Work out the finished part from the listing and answer in its coordinate system (mm). Face numbers are marked on the shaded views. A direction names the side the tool comes from. Give positions to 0.01 mm unless a question says otherwise; leave off trailing zeros. Loops run counter-clockwise (first coordinate to the right, second up) from the corner with the lowest first, then second, coordinate; pieces in that order, holes last. Notation, with made-up numbers: (14.25, 59.25) - (41.25, 59.25) arc R23 ccw to (41.25, 70.25) - close; hole circle Ø10 at (59.25, -8.5). An arc over 180 degrees is marked (long way). One line per question, with ' | ' between items. Start each with the question number.
1. For a pull along Z with two mould halves and no side action, classify the marked faces 6, 7 and 8 as released by +Z, released by -Z, zero draft, split by the parting line, or undercut.
2. Which of the six approach directions +Z, -Z, +X, -X, +Y, -Y give full straight-line access (tool end or side, diameter ignored) to the marked faces 1, 2, 3, 4 and 5?
3. Find the intervals of material crossed by line 1 (Z direction, x = 2, y = 0.5); line 2 (X direction, y = 0.6, z = 2); line 3 (Z direction, x = 37.5, y = -0.25), in increasing order.
4. Section B-B (y = 3.25) is taken. Determine the outline of the cut face in (x, z).
5. Section A-A (z = 10) is taken. Determine the outline of the cut face in (x, y).
6. Each of these flat-tipped pins is pushed along its axis until it touches: pin 1 (12 mm diameter, centred on x = 41.5, z = 11.5, fed in from -Y); pin 2 (1.5 mm diameter, centred on y = 1.5, z = 7.5, fed in from +X); pin 3 (0.7 mm diameter, centred on x = 16.5, y = -6, fed in from +Z); pin 4 (2 mm diameter, centred on x = 25.5, z = 1, fed in from -Y). Where does it stop, or does it pass through?
7. Section C-C (y = -4.25) is taken. Give the number of separate pieces and of enclosed holes in the cut face, plus the area to 3 significant figures.
from build123d import *

# Parameters (mm, degrees)
SKETCH1_W           = 48.3
SKETCH1_H           = 25.5
SKETCH1_R           = 1.5
BOSS_EXTRUDE1_DEPTH = 4.4
FILLET1_R           = 2
SKETCH2_W           = 2.54
SKETCH2_H           = 2.54
BOSS_EXTRUDE2_DEPTH = 2.35
SKETCH3_W           = 0.66
SKETCH3_H           = 0.66
BOSS_EXTRUDE3_DEPTH = 5.33
SKETCH4_W           = 3.4
SKETCH4_H           = 7.5
CUT_EXTRUDE1_DEPTH  = 0.7
SKETCH5_W           = 7.5
SKETCH5_H           = 3.7
BOSS_EXTRUDE4_DEPTH = 0.3
SKETCH6_W           = 7.4
SKETCH6_H           = 16.14
CUT_EXTRUDE2_DEPTH  = 2.4
SKETCH7_W           = 4
SKETCH7_H           = 4
CUT_EXTRUDE3_DEPTH  = 3.3


with BuildPart() as part:
    # Sketch1 → Boss-Extrude1 (new body)
    with BuildSketch(Plane(origin=(0, 0, 0), x_dir=(1, 0, 0), z_dir=(0, 1, 0))):
        with Locations((24.15, -12.75)):
            Rectangle(SKETCH1_W, SKETCH1_H)
        with Locations((46.3, -2)):
            Circle(SKETCH1_R, mode=Mode.SUBTRACT)
        with Locations((2, -2)):
            Circle(SKETCH1_R, mode=Mode.SUBTRACT)
        with Locations((46.3, -23.5)):
            Circle(SKETCH1_R, mode=Mode.SUBTRACT)
        with Locations((2, -23.5)):
            Circle(SKETCH1_R, mode=Mode.SUBTRACT)
    extrude(amount=BOSS_EXTRUDE1_DEPTH)

    # Fillet1
    fillet1_edges = [part.edges().sort_by_distance(p)[0] for p in [
        (48.3, 2.2, 25.5),
        (0, 2.2, 25.5),
        (0, 2.2, 0),
        (48.3, 2.2, 0),
    ]]
    fillet(fillet1_edges, radius=FILLET1_R)

    # Sketch2 → Boss-Extrude2 (add)
    with BuildSketch(Plane.XZ):
        with Locations((6.37, 24.23)):
            Rectangle(SKETCH2_W, SKETCH2_H)
        with Locations((8.91, 24.23)):
            Rectangle(SKETCH2_W, SKETCH2_H)
        with Locations((11.45, 24.23)):
            Rectangle(SKETCH2_W, SKETCH2_H)
        with Locations((13.99, 24.23)):
            Rectangle(SKETCH2_W, SKETCH2_H)
        with Locations((16.53, 24.23)):
            Rectangle(SKETCH2_W, SKETCH2_H)
        with Locations((19.07, 24.23)):
            Rectangle(SKETCH2_W, SKETCH2_H)
        with Locations((21.61, 24.23)):
            Rectangle(SKETCH2_W, SKETCH2_H)
        with Locations((24.15, 24.23)):
            Rectangle(SKETCH2_W, SKETCH2_H)
        with Locations((26.69, 24.23)):
            Rectangle(SKETCH2_W, SKETCH2_H)
        with Locations((29.23, 24.23)):
            Rectangle(SKETCH2_W, SKETCH2_H)
        with Locations((31.77, 24.23)):
            Rectangle(SKETCH2_W, SKETCH2_H)
        with Locations((34.31, 24.23)):
            Rectangle(SKETCH2_W, SKETCH2_H)
        with Locations((36.85, 24.23)):
            Rectangle(SKETCH2_W, SKETCH2_H)
        with Locations((39.39, 24.23)):
            Rectangle(SKETCH2_W, SKETCH2_H)
        with Locations((41.93, 24.23)):
            Rectangle(SKETCH2_W, SKETCH2_H)
        with Locations((41.93, 1.27)):
            Rectangle(SKETCH2_W, SKETCH2_H)
        with Locations((39.39, 1.27)):
            Rectangle(SKETCH2_W, SKETCH2_H)
        with Locations((36.85, 1.27)):
            Rectangle(SKETCH2_W, SKETCH2_H)
        with Locations((34.31, 1.27)):
            Rectangle(SKETCH2_W, SKETCH2_H)
        with Locations((31.77, 1.27)):
            Rectangle(SKETCH2_W, SKETCH2_H)
        with Locations((29.23, 1.27)):
            Rectangle(SKETCH2_W, SKETCH2_H)
        with Locations((26.69, 1.27)):
            Rectangle(SKETCH2_W, SKETCH2_H)
        with Locations((24.15, 1.27)):
            Rectangle(SKETCH2_W, SKETCH2_H)
        with Locations((21.61, 1.27)):
            Rectangle(SKETCH2_W, SKETCH2_H)
        with Locations((19.07, 1.27)):
            Rectangle(SKETCH2_W, SKETCH2_H)
        with Locations((16.53, 1.27)):
            Rectangle(SKETCH2_W, SKETCH2_H)
        with Locations((13.99, 1.27)):
            Rectangle(SKETCH2_W, SKETCH2_H)
        with Locations((11.45, 1.27)):
            Rectangle(SKETCH2_W, SKETCH2_H)
        with Locations((8.91, 1.27)):
            Rectangle(SKETCH2_W, SKETCH2_H)
        with Locations((6.37, 1.27)):
            Rectangle(SKETCH2_W, SKETCH2_H)
    extrude(amount=BOSS_EXTRUDE2_DEPTH)

    # Sketch3 → Boss-Extrude3 (add)
    with BuildSketch(Plane.XZ.offset(2.35)):
        with Locations((6.37, 24.23)):
            Rectangle(SKETCH3_W, SKETCH3_H)
        with Locations((8.91, 24.23)):
            Rectangle(SKETCH3_W, SKETCH3_H)
        with Locations((11.45, 24.23)):
            Rectangle(SKETCH3_W, SKETCH3_H)
        with Locations((13.99, 24.23)):
            Rectangle(SKETCH3_W, SKETCH3_H)
        with Locations((16.53, 24.23)):
            Rectangle(SKETCH3_W, SKETCH3_H)
        with Locations((19.07, 24.23)):
            Rectangle(SKETCH3_W, SKETCH3_H)
        with Locations((21.61, 24.23)):
            Rectangle(SKETCH3_W, SKETCH3_H)
        with Locations((24.15, 24.23)):
            Rectangle(SKETCH3_W, SKETCH3_H)
        with Locations((26.69, 24.23)):
            Rectangle(SKETCH3_W, SKETCH3_H)
        with Locations((29.23, 24.23)):
            Rectangle(SKETCH3_W, SKETCH3_H)
        with Locations((31.77, 24.23)):
            Rectangle(SKETCH3_W, SKETCH3_H)
        with Locations((34.31, 24.23)):
            Rectangle(SKETCH3_W, SKETCH3_H)
        with Locations((36.85, 24.23)):
            Rectangle(SKETCH3_W, SKETCH3_H)
        with Locations((39.39, 24.23)):
            Rectangle(SKETCH3_W, SKETCH3_H)
        with Locations((41.93, 24.23)):
            Rectangle(SKETCH3_W, SKETCH3_H)
        with Locations((41.93, 1.27)):
            Rectangle(SKETCH3_W, SKETCH3_H)
        with Locations((39.39, 1.27)):
            Rectangle(SKETCH3_W, SKETCH3_H)
        with Locations((36.85, 1.27)):
            Rectangle(SKETCH3_W, SKETCH3_H)
        with Locations((34.31, 1.27)):
            Rectangle(SKETCH3_W, SKETCH3_H)
        with Locations((31.77, 1.27)):
            Rectangle(SKETCH3_W, SKETCH3_H)
        with Locations((29.23, 1.27)):
            Rectangle(SKETCH3_W, SKETCH3_H)
        with Locations((26.69, 1.27)):
            Rectangle(SKETCH3_W, SKETCH3_H)
        with Locations((24.15, 1.27)):
            Rectangle(SKETCH3_W, SKETCH3_H)
        with Locations((21.61, 1.27)):
            Rectangle(SKETCH3_W, SKETCH3_H)
        with Locations((19.07, 1.27)):
            Rectangle(SKETCH3_W, SKETCH3_H)
        with Locations((16.53, 1.27)):
            Rectangle(SKETCH3_W, SKETCH3_H)
        with Locations((13.99, 1.27)):
            Rectangle(SKETCH3_W, SKETCH3_H)
        with Locations((11.45, 1.27)):
            Rectangle(SKETCH3_W, SKETCH3_H)
        with Locations((8.91, 1.27)):
            Rectangle(SKETCH3_W, SKETCH3_H)
        with Locations((6.37, 1.27)):
            Rectangle(SKETCH3_W, SKETCH3_H)
    extrude(amount=BOSS_EXTRUDE3_DEPTH)

    # Sketch4 → Cut-Extrude1 (cut)
    with BuildSketch(Plane(origin=(0, 4.4, 0), x_dir=(1, 0, 0), z_dir=(0, 1, 0))):
        with Locations((46.6, -12.75)):
            Rectangle(SKETCH4_W, SKETCH4_H)
    extrude(amount=-CUT_EXTRUDE1_DEPTH, mode=Mode.SUBTRACT)

    # Sketch5 → Boss-Extrude4 (add)
    with BuildSketch(Plane(origin=(48.3, 0, 0), x_dir=(0, 0, -1), z_dir=(1, 0, 0))):
        with Locations((-12.75, 1.85)):
            Rectangle(SKETCH5_W, SKETCH5_H)
    extrude(amount=BOSS_EXTRUDE4_DEPTH)

    # Sketch6 → Cut-Extrude2 (cut)
    with BuildSketch(Plane(origin=(0, 4.4, 0), x_dir=(1, 0, 0), z_dir=(0, 1, 0))):
        with Locations((3.7, -12.75)):
            Rectangle(SKETCH6_W, SKETCH6_H)
    extrude(amount=-CUT_EXTRUDE2_DEPTH, mode=Mode.SUBTRACT)

    # Sketch7 → Cut-Extrude3 (cut)
    with BuildSketch(Plane(origin=(0, 4.4, 0), x_dir=(1, 0, 0), z_dir=(0, 1, 0))):
        with Locations((2, -2)):
            Rectangle(SKETCH7_W, SKETCH7_H)
        with Locations((46.3, -2)):
            Rectangle(SKETCH7_W, SKETCH7_H)
        with Locations((46.3, -23.5)):
            Rectangle(SKETCH7_W, SKETCH7_H)
        with Locations((2, -23.5)):
            Rectangle(SKETCH7_W, SKETCH7_H)
    extrude(amount=-CUT_EXTRUDE3_DEPTH, mode=Mode.SUBTRACT)


solid = part.part
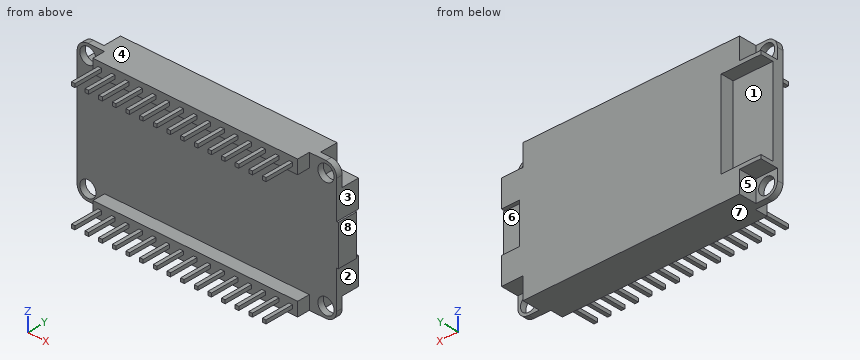
Conclusion:
1) face 6: undercut | face 7: released by -Z | face 8: zero draft
2) face 1: -X, +Y | face 2: -Z, +X, +Y, -Y | face 3: +Z, +X, +Y, -Y | face 4: +Z, +X, -X, +Y, -Y | face 5: -Z, -X, +Y
3) line 1: 0 to 0.5, 3.5 to 22, 25 to 25.5 | line 2: 0 to 0.5, 3.5 to 44.8, 47.8 to 48.3 | line 3: 0 to 2.54, 22.96 to 25.5
4) outline: (0, 4) - (4, 4) - (4, 0) - (44.3, 0) - (44.3, 4) - (48.3, 4) - (48.3, 9) - (48.6, 9) - (48.6, 16.5) - (48.3, 16.5) - (48.3, 21.5) - (44.3, 21.5) - (44.3, 25.5) - (4, 25.5) - (4, 21.5) - (0, 21.5) - (0, 20.82) - (7.4, 20.82) - (7.4, 4.68) - (0, 4.68) - close
5) outline: (0, 0) - (48.6, 0) - (48.6, 3.7) - (44.9, 3.7) - (44.9, 4.4) - (7.4, 4.4) - (7.4, 2) - (0, 2) - close
6) pin 1: y = 0 | pin 2: x = 48.3 | pin 3: z = 24.56 | pin 4: y = -7.68
7) separate pieces: 30 | enclosed holes: 0 | area: 13.1 mm²
